Autodesk Inventor part; units mm, degrees
ref_plane "YZ Plane" through (0, 0, 0) normal (1, 0, 0) x (0, 1, 0)
ref_plane "XZ Plane" through (0, 0, 0) normal (0, 1, 0) x (-1, 0, 0)
ref_plane "XY Plane" through (0, 0, 0) normal (0, 0, 1) x (1, 0, 0)
sketch "Szkic2" plane through (0, 0, 0) normal (1, 0, 0) x (0, 1, 0)
  line L0 (0, -2.9) -> (0, 2.9)
  line L1 (-1.5, -1.5) -> (-1.5, 1.5)
  line L2 (-1.5, -1.5) -> (0, -2.9)
  line L3 (-1.5, 1.5) -> (0, 2.9)
  line L4 (0, 0) -> (-40, 0)
  line L5 (-40, 0) -> (-40, -1.5)
  line L6 (-40, -1.5) -> (-1.5, -1.5)
  dimension "d0" = 5.8
  dimension "d2" = 3
  dimension "d3" = 1.5
  dimension "d4" = 40
  dimension "d5" = 1.5
revolve "Obrót1" add sketch "Szkic2" angle 360 about axis through (0, 0, 0) along (0, -1, 0) contours L2 L1 L4 L0 | L6 L5 L4 L1
sketch "Szkic3" plane through (0, 0, 0) normal (0, 1, 0) x (1, 0, 0)
  line L0 (-1.1673, -0.633) -> (-1.1318, 0.6945)
  line L1 (-1.1318, 0.6945) -> (0.0355, 1.3274)
  line L2 (0.0355, 1.3274) -> (1.1673, 0.633)
  line L3 (1.1673, 0.633) -> (1.1318, -0.6945)
  line L4 (1.1318, -0.6945) -> (-0.0355, -1.3274)
  line L5 (-0.0355, -1.3274) -> (-1.1673, -0.633)
  point P0 (0, 0)
  point P1 (0, 0)
  dimension "d7" = 2.3
extrude "Wyciągnięcie proste1" cut sketch "Szkic3" against normal blind 2
fillet "Zaokrąglenie1" radius 0.5 6 edges at (-1.1496, -2, -0.0308) (-0.6014, -2, 0.9802) (-0.5482, -2, -1.011) (0.6014, -2, -0.9802) (0.5482, -2, 1.011) (1.1496, -2, 0.0308)
fillet "Zaokrąglenie2" radius 0.5 1 edges at (0, -1.5, 1.5)
fillet "Zaokrąglenie3" radius 0.1 1 edges at (0, 0, 2.9)
thread "Gwint1"
chamfer "Faza1" distance 0.5 angle 45 1 edges at (0, -40, 1.5)
properties part number "Screw M3 40mm flat head"
Design review of the part built by this model. Coordinates are the model's own, in mm. A direction names the side the tool comes from. Give positions to 0.01 mm unless a question says otherwise; leave off trailing zeros. Write each loop counter-clockwise with the first axis right and the second up, starting at its lowest first coordinate (ties: lowest second). Pieces come first, ordered by that corner, then holes. Notation, with made-up numbers: M 65.25,-8.75 L 115.25,-8.75 A20 ccw 115.25,2.25 Z; hole C 30,76.25 d10. An arc over 180 degrees is marked long. Answer as a JSON object with one key per item and string values. Group by question number.
1) We need section A-A (y = -32). Give the boundary of the cut face in (x, z), and give its area (3 significant figures).
2) Tool access review of faces 4 (the face through (-1, 0, -1)), 5 (the face through (0.593, -0.74, -0.985)): name each direction out of +Z, -Z, +X, -X, +Y, -Y from which nothing blocks a thin tool from reaching the whole face with its end or side.
3) Clearance check with flat-ended pins moving along their axes: pin 1 Ø1 at (x, y) = (0, -19.5) entering from -Z; pin 2 Ø1.5 at (x, z) = (2, -1.5) entering from +Y; pin 3 Ø0.7 at (x, z) = (0, 0) entering from +Y. State where each tip first meets the part, or that it passes through.
4) For line 1 along Y through (x, z) = (-0.2, 0); line 2 along X through (y, z) = (-4.5, 0.1); line 3 along Z through (x, y) = (0.95, -15), list the stretches that pass through material, from the lowest coordinate up.
5) Mouldability with a two-part tool opening along X and no side actions: class faces 1 (the face through (0, -40, 0)), 2 (the face through (-0.07, -20.33, 1.5)), 3 (the face through (0.556, -0.74, 1.007)) as released by +X, released by -X, zero draft, split by the parting line, or undercut.
Answer key:
{
 "1": {"outline": "C 0,0 d3", "area": "7.07 mm²"},
 "2": {"face 4": "+Z, -Z, +X, -X, +Y", "face 5": "+Y"},
 "3": {"pin 1": "stops at z = -1.5", "pin 2": "stops at y = 0", "pin 3": "stops at y = -2"},
 "4": {"line 1": "y = -40 to -2", "line 2": "x = -1.5 to 1.5", "line 3": "z = -1.16 to 1.16"},
 "5": {"face 1": "zero draft", "face 2": "split by the parting line", "face 3": "undercut"}
}
